from build123d import *

# Parameters (mm, degrees)
BOSS_EXTRUDE1_DEPTH        = 3.175
F_9_0_196_DIAMETER_HOLE1_D = 4.9784


with BuildPart() as part:
    # Sketch1 → Boss-Extrude1 (new body)
    with BuildSketch(Plane(origin=(0, 0, 0), x_dir=(0, 1, 0), z_dir=(0, 0, 1))):
        Polygon((-80.9625, -12.7), (-80.9625, -38.1), (-106.3625, -38.1), (-106.3625, 12.7), (20.6375, 12.7), (20.6375, 114.3), (46.0375, 114.3), (46.0375, 12.7), (106.3625, 12.7), (106.3625, -38.1), (20.6375, -38.1), (20.6375, -12.7), align=None)
    extrude(amount=BOSS_EXTRUDE1_DEPTH)

    # #9 (0.196) Diameter Hole1 (through all)
    with Locations(Plane.XY.offset(3.175)):
        with Locations((25.4, -93.6625), (-153.251995768, -35.15541816), (-101.6, 33.3375), (-174.461563536, 15.375329004)):
            Hole(F_9_0_196_DIAMETER_HOLE1_D / 2)


solid = part.part
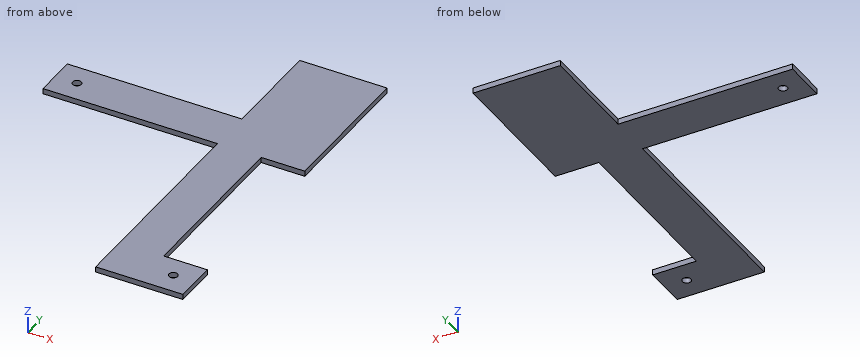
Geometry: final body of the model. Coordinates: model frame, mm. Give positions to 0.01 mm unless a question says otherwise; leave off trailing zeros. Write each loop counter-clockwise with the first axis right and the second up, starting at its lowest first coordinate (ties: lowest second). Pieces come first, ordered by that corner, then holes.
(1) Cut plane D-D, the plane y = 59. Return loops of the section in (x, z) (3 decimals), then the cut area to 3 significant figures.
(2) Cut plane A-A, the plane x = -101.6. Return loops of the section in (y, z) (1 decimal).
(3) Cut plane B-B, the plane x = 25.4. Return loops of the section in (y, z) (1 decimal), then the cut area to 3 significant figures.
(4) First-contact query: P1, Ø1.5, axis at y = -39.5, z = 2.5, coming from the -X side; P2, Ø1.5, axis at x = -45.5, z = 1.5, coming from the +Y side. Flat tips, straight axial feed; report the tip coordinate or a pass-through.
(5) Cut plane C-C, the plane z = 1.1. Return loops of the section in (x, y), then the cut area to 3 significant figures.
(6) Ray query, line 1 (Y direction, x = 25.4, z = 2.3); line 2 (Y direction, x = 15.5, z = 1.35); line 3 (Y direction, x = -101.6, z = 1.6). Return the intervals inside material, ascending.
Values follow:
1. outline: (-12.7, 0) - (38.1, 0) - (38.1, 3.175) - (-12.7, 3.175) - close
1. area: 161 mm2
2. outline: (20.6, 0) - (30.8, 0) - (30.8, 3.2) - (20.6, 3.2) - close; (35.8, 0) - (46, 0) - (46, 3.2) - (35.8, 3.2) - close
3. outline: (-106.4, 0) - (-96.2, 0) - (-96.2, 3.2) - (-106.4, 3.2) - close; (-91.2, 0) - (-81, 0) - (-81, 3.2) - (-91.2, 3.2) - close; (20.6, 0) - (106.4, 0) - (106.4, 3.2) - (20.6, 3.2) - close
3. area: 337 mm2
4. P1: stops at x = -12.7
4. P2: stops at y = 46.04
5. outline: (-114.3, 20.64) - (-12.7, 20.64) - (-12.7, -106.36) - (38.1, -106.36) - (38.1, -80.96) - (12.7, -80.96) - (12.7, 20.64) - (38.1, 20.64) - (38.1, 106.36) - (-12.7, 106.36) - (-12.7, 46.04) - (-114.3, 46.04) - close; hole circle Ø4.98 at (-101.6, 33.34); hole circle Ø4.98 at (25.4, -93.66)
5. area: 10,800 mm2
6. line 1: y = -106.36 to -96.15, -91.17 to -80.96, 20.64 to 106.36
6. line 2: y = -106.36 to -80.96, 20.64 to 106.36
6. line 3: y = 20.64 to 30.85, 35.83 to 46.04
